```python
from build123d import *

# Parameters (mm, degrees)
SKETCH_1_R      = 30
SKETCH_1_R_2    = 25
SKETCH_1_R_3    = 10
SKETCH_1_R_4    = 1
SKETCH_1_R_5    = 6
EXTRUDE_1_DEPTH = 3


with BuildPart() as part:
    # 草图1 → 凸台-拉伸1 (new body)
    # profile 1 of 6: a face of its own
    with BuildSketch(Plane(origin=(0, 0, 0), x_dir=(1, 0, 0), z_dir=(0, 1, 0))):
        with Locations(Location((0, 0, 0), (0, 0, 270))):
            Circle(SKETCH_1_R)
        Circle(SKETCH_1_R_2, mode=Mode.SUBTRACT)
    # profile 2 of 6: a face of its own
    with BuildSketch(Plane(origin=(0, 0, 0), x_dir=(1, 0, 0), z_dir=(0, 1, 0))):
        with BuildLine():
            ThreePointArc((-9.921567416, -1.25), (-10, 0), (-9.921567416, 1.25))
            Line((-9.921567416, 1.25), (-24.968730444, 1.25))
            ThreePointArc((-24.968730444, 1.25), (-25, 0), (-24.968730444, -1.25))
            Line((-24.968730444, -1.25), (-9.921567416, -1.25))
        make_face()
    # profile 3 of 6: a face of its own
    with BuildSketch(Plane(origin=(0, 0, 0), x_dir=(1, 0, 0), z_dir=(0, 1, 0))):
        with BuildLine():
            ThreePointArc((-1.25, 9.921567416), (0, 10), (1.25, 9.921567416))
            Line((1.25, 9.921567416), (1.25, 24.968730444))
            ThreePointArc((1.25, 24.968730444), (0, 25), (-1.25, 24.968730444))
            Line((-1.25, 24.968730444), (-1.25, 9.921567416))
        make_face()
    # profile 4 of 6: a face of its own
    with BuildSketch(Plane(origin=(0, 0, 0), x_dir=(1, 0, 0), z_dir=(0, 1, 0))):
        Circle(SKETCH_1_R_3)
        with Locations(Location((8, 0, 0), (0, 0, 270))):
            Circle(SKETCH_1_R_4, mode=Mode.SUBTRACT)
        with Locations(Location((0, -8, 0), (0, 0, 270))):
            Circle(SKETCH_1_R_4, mode=Mode.SUBTRACT)
        with Locations(Location((-8, 0, 0), (0, 0, 270))):
            Circle(SKETCH_1_R_4, mode=Mode.SUBTRACT)
        with Locations(Location((0, 8, 0), (0, 0, 270))):
            Circle(SKETCH_1_R_4, mode=Mode.SUBTRACT)
        with Locations(Location((0, 0, 0), (0, 0, 270))):
            Circle(SKETCH_1_R_5, mode=Mode.SUBTRACT)
    # profile 5 of 6: a face of its own
    with BuildSketch(Plane(origin=(0, 0, 0), x_dir=(1, 0, 0), z_dir=(0, 1, 0))):
        with BuildLine():
            Line((24.968730444, 1.25), (9.921567416, 1.25))
            ThreePointArc((9.921567416, 1.25), (9.980372592, 0.626229125), (10, 0))
            ThreePointArc((10, 0), (9.980372592, -0.626229125), (9.921567416, -1.25))
            Line((9.921567416, -1.25), (24.968730444, -1.25))
            ThreePointArc((24.968730444, -1.25), (24.992181388, -0.625195526), (25, 0))
            ThreePointArc((25, 0), (24.992181388, 0.625195526), (24.968730444, 1.25))
        make_face()
    # profile 6 of 6: a face of its own
    with BuildSketch(Plane(origin=(0, 0, 0), x_dir=(1, 0, 0), z_dir=(0, 1, 0))):
        with BuildLine():
            Line((1.25, -24.968730444), (1.25, -9.921567416))
            ThreePointArc((1.25, -9.921567416), (0, -10), (-1.25, -9.921567416))
            Line((-1.25, -9.921567416), (-1.25, -24.968730444))
            ThreePointArc((-1.25, -24.968730444), (0, -25), (1.25, -24.968730444))
        make_face()
    extrude(amount=EXTRUDE_1_DEPTH)


solid = part.part
```
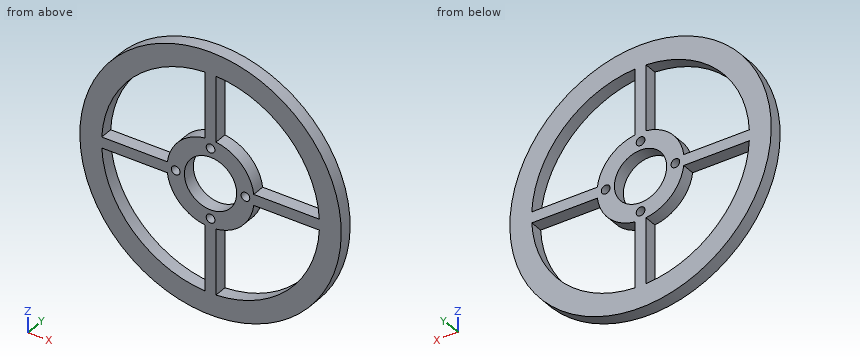
The model under review builds one solid part; all positions refer to its coordinate system, in mm. Round coordinates to 2 decimals unless told otherwise and drop trailing zeros. Loops run counter-clockwise (first coordinate to the right, second up) from the corner with the lowest first, then second, coordinate; pieces in that order, holes last.
1) Wall thickness on line 1 along X through (y, z) = (1.9, 0); line 2 along X through (y, z) = (2.15, 1.5); line 3 along X through (y, z) = (1.15, 22): over which ranges is each line inside the solid? List them lowest first.
Values follow:
line 1: x = -30 to -9, -7 to -6, 6 to 7, 9 to 30
line 2: x = -29.96 to -24.95, -9.89 to -5.81, 5.81 to 9.89, 24.95 to 29.96
line 3: x = -20.4 to -11.87, -1.25 to 1.25, 11.87 to 20.4
2) Consider section A-A on x = 0. State the section outline as (y, z) points.
Values follow:
outline: (0, -30) - (3, -30) - (3, -9) - (0, -9) - close; (0, -7) - (3, -7) - (3, -6) - (0, -6) - close; (0, 6) - (3, 6) - (3, 7) - (0, 7) - close; (0, 9) - (3, 9) - (3, 30) - (0, 30) - close
3) Consider section C-C on z = 2. State the section outline as (x, y) points.
Values follow:
outline: (-29.93, 0) - (-24.92, 0) - (-24.92, 3) - (-29.93, 3) - close; (-9.8, 0) - (-5.66, 0) - (-5.66, 3) - (-9.8, 3) - close; (5.66, 0) - (9.8, 0) - (9.8, 3) - (5.66, 3) - close; (24.92, 0) - (29.93, 0) - (29.93, 3) - (24.92, 3) - close
4) Consider section D-D on z = -13. State the section outline as (x, y) points.
Values follow:
outline: (-27.04, 0) - (-21.35, 0) - (-21.35, 3) - (-27.04, 3) - close; (-1.25, 0) - (1.25, 0) - (1.25, 3) - (-1.25, 3) - close; (21.35, 0) - (27.04, 0) - (27.04, 3) - (21.35, 3) - close
5) Clearance check with flat-ended pins moving along their axes: P1, Ø0.9, axis at y = 1.5, z = -19, coming from the -X side; P2, Ø1.5, axis at x = -13.5, y = 2, coming from the +Z side; P3, Ø1.5, axis at y = 1.5, z = -19, coming from the +X side. State where each tip first meets the part, or that it passes through.
Values follow:
P1: stops at x = -23.58
P2: stops at z = 27.16
P3: stops at x = 23.81
6) Consider section B-B on y = 1.85. Give the number of separate pieces and of enclosed holes in the cut face, then the cut area to 3 significant figures.
Values follow:
separate pieces: 1
enclosed holes: 9
area: 1,200 mm2
